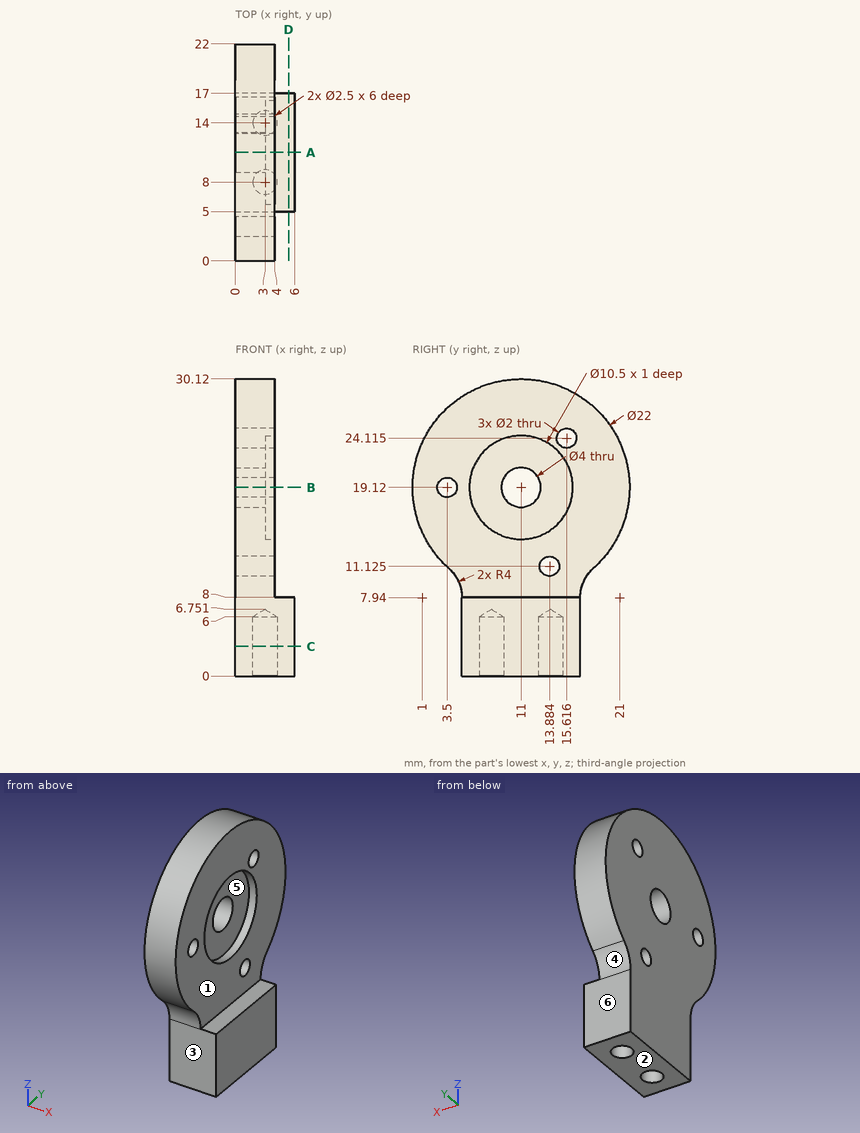
Answer from the drawing. Dimensions are ordinates in mm from the lowest x, y and z of the part. A direction names the side the tool comes from. Coordinates: 2 decimals unless noted, no trailing zeros. Order: outer loops, then holes, each group sorted by start corner. A loop starts at its lowest first (then second) coordinate and runs counter-clockwise, first axis right, second up. Notation, with made-up numbers: (-31.5, 82.5) -> (8.5, 82.5) arc R36 cw to (8.5, 121.5) -> close; hole circle Ø5 at (-5.75, -34.5). An arc over 180 degrees is marked (long way). Answer as a JSON object with one key per item and string values.
1) Each of these flat-tipped pins is pushed along its axis until it touches: pin 1 (1.8 mm diameter, centred on x = 1.5, z = 3.5, fed in from +Y); pin 2 (8.5 mm diameter, centred on y = 11, z = 21.5, fed in from +X); pin 3 (1.5 mm diameter, centred on y = 18.5, z = 26.5, fed in from -X); pin 4 (4.5 mm diameter, centred on y = 11, z = 19.12, fed in from +X). Where does it stop, or does it pass through?
Model answer:
{"pin 1": "stops at y = 17", "pin 2": "stops at x = 4", "pin 3": "stops at x = 0", "pin 4": "stops at x = 3"}
2) A cutting plane is placed at B-B, the plane z = 19.12. Determine the outline of the cut face in (x, y).
Model answer:
{"outline": "(0, 0) -> (4, 0) -> (4, 2.5) -> (0, 2.5) -> close; (0, 4.5) -> (4, 4.5) -> (4, 5.75) -> (3, 5.75) -> (3, 9) -> (0, 9) -> close; (0, 13) -> (3, 13) -> (3, 16.25) -> (4, 16.25) -> (4, 22) -> (0, 22) -> close"}
3) A cutting plane is placed at C-C, the plane z = 3. Determine the outline of the cut face in (x, y).
Model answer:
{"outline": "(0, 5) -> (6, 5) -> (6, 17) -> (0, 17) -> close; hole circle Ø2.5 at (3, 8); hole circle Ø2.5 at (3, 14)"}
4) A tool of negligible diameter and unlimited length cuts with its end or side. For the marked faces 1, 2 and 3, from which of +Z, -Z, +X, -X, +Y, -Y can it reach the whole face along a straight path? Write none if from no direction.
Model answer:
{"face 1": "+Z, +X, +Y, -Y", "face 2": "-Z, +X, -X, +Y, -Y", "face 3": "-Z, +X, -X, -Y"}
5) A cutting plane is placed at D-D, the plane x = 5.4. Determine the outline of the cut face in (y, z), plus the area to 3 significant figures.
Model answer:
{"outline": "(5, 0) -> (17, 0) -> (17, 7.94) arc R4 cw to (17, 8) -> (5, 8) arc R4 cw to (5, 7.94) -> close", "area": "96.0 mm²"}
6) A cutting plane is placed at A-A, the plane y = 11. Determine the outline of the cut face in (x, z).
Model answer:
{"outline": "(0, 0) -> (6, 0) -> (6, 8) -> (4, 8) -> (4, 13.87) -> (3, 13.87) -> (3, 17.12) -> (0, 17.12) -> close; (0, 21.12) -> (3, 21.12) -> (3, 24.37) -> (4, 24.37) -> (4, 30.12) -> (0, 30.12) -> close"}
7) The mould has two halves that part along Z. Classify the marked faces 4, 5 and 6: released by +Z, released by -Z, zero draft, split by the parting line, or undercut.
Model answer:
{"face 4": "released by -Z", "face 5": "undercut", "face 6": "zero draft"}
8) Consider line 1 along Y through (x, z) = (3, 4.65); line 2 along X through (y, z) = (14, 4.6); line 3 along X through (y, z) = (7.75, 19). Determine where each line is inside the solid, lowest interval first. Write a range as from..to.
Model answer:
{"line 1": "y = 5..6.75, 9.25..12.75, 15.25..17", "line 2": "x = 0..1.75, 4.25..6", "line 3": "x = 0..3"}
